Can you work these out from the model? Positions are in its coordinate system, mm. A direction names the side the tool comes from. Coordinates: 2 decimals unless noted, no trailing zeros. Order: outer loops, then holes, each group sorted by start corner. A loop starts at its lowest first (then second) coordinate and runs counter-clockwise, first axis right, second up. Notation, with made-up numbers: (-38.5, 15) -> (-26.5, 15) arc R15 cw to (-26.5, 32) -> close; hole circle Ø7 at (-23, -30). An arc over 180 degrees is marked (long way). Answer in a Markdown table with one row per item.
```python
from build123d import *

# Parameters (mm, degrees)
BOSS_EXTRUDE1_DEPTH = 45
SKETCH3_W           = 92.200496998
SKETCH3_H           = 5.5
BOSS_EXTRUDE2_DEPTH = 1
SKETCH4_R           = 2.5
CUT_EXTRUDE2_DEPTH  = 7.222605
SKETCH8_R           = 4.5
CUT_EXTRUDE7_DEPTH  = 0.386255
CUT_EXTRUDE3_START  = -13.60831
SKETCH5_R           = 2.5
CUT_EXTRUDE3_DEPTH  = 13.60831
CUT_EXTRUDE5_START  = -14
SKETCH6_R           = 4.25
CUT_EXTRUDE5_DEPTH  = 1.7
SKETCH10_R          = 2.6
CUT_EXTRUDE8_DEPTH  = 32
SKETCH11_R          = 10
BOSS_EXTRUDE3_DEPTH = 1
CUT_EXTRUDE10_DEPTH = 46.0000001


with BuildPart() as part:
    # Sketch1 → Boss-Extrude1 (new body)
    with BuildSketch(Plane(origin=(0, 0, 0), x_dir=(1, 0, 0), z_dir=(0, 1, 0))):
        with BuildLine():
            Line((67.073634163, -66.174942219), (25, 6.698729811))
            Line((25, 6.698729811), (43.49555567, 17.377143855))
            ThreePointArc((43.49555567, 17.377143855), (0, 32), (-43.49555567, 17.377143855))
            Line((-43.49555567, 17.377143855), (-25, 6.698729811))
            Line((-25, 6.698729811), (-67.073634163, -66.174942219))
            Line((-67.073634163, -66.174942219), (-71.100248499, -73.149242831))
            Line((-71.100248499, -73.149242831), (-63.915003714, -73.149242831))
            Line((-63.915003714, -73.149242831), (-48.529056191, -46.5))
            ThreePointArc((-48.529056191, -46.5), (-46.698929172, -44.669872981), (-44.198929172, -44))
            Line((-44.198929172, -44), (44.198929172, -44))
            ThreePointArc((44.198929172, -44), (46.698929172, -44.669872981), (48.529056191, -46.5))
            Line((48.529056191, -46.5), (63.915003714, -73.149242831))
            Line((63.915003714, -73.149242831), (71.100248499, -73.149242831))
            Line((71.100248499, -73.149242831), (67.073634163, -66.174942219))
        make_face()
        Polygon((-20, 20), (-13, 20), (-13, 18), (-7, 18), (-7, 20), (7, 20), (7, 18), (13, 18), (13, 20), (20, 20), (20, 13), (18, 13), (18, 7), (20, 7), (20, 0), (-20, 0), (-20, 7), (-18, 7), (-18, 13), (-20, 13), align=None, mode=Mode.SUBTRACT)
        with BuildLine():
            Line((-27.744446501, -15.5), (27.744446501, -15.5))
            ThreePointArc((27.744446501, -15.5), (30.244446501, -16.169872981), (32.074573519, -18))
            Line((32.074573519, -18), (39.580127019, -31))
            ThreePointArc((39.580127019, -31), (39.580127019, -36), (35.25, -38.5))
            Line((35.25, -38.5), (-35.25, -38.5))
            ThreePointArc((-35.25, -38.5), (-39.580127019, -36), (-39.580127019, -31))
            Line((-39.580127019, -31), (-32.074573519, -18))
            ThreePointArc((-32.074573519, -18), (-30.244446501, -16.169872981), (-27.744446501, -15.5))
        make_face(mode=Mode.SUBTRACT)
    extrude(amount=BOSS_EXTRUDE1_DEPTH)

    # Sketch3 → Boss-Extrude2 (add)
    with BuildSketch(Plane(origin=(21.650635095, 0, -12.5), x_dir=(-0.5, 0, -0.866025404), z_dir=(0.866025404, 0, -0.5))):
        with Locations((-52.79897831, 32.25)):
            Rectangle(SKETCH3_W, SKETCH3_H)
        with Locations((-52.79897831, 12.75)):
            Rectangle(SKETCH3_W, SKETCH3_H)
    boss_extrude2 = extrude(amount=BOSS_EXTRUDE2_DEPTH)

    # Sketch4 → Cut-Extrude2 (cut)
    with BuildSketch(Plane(origin=(22.516660498, 0, -13), x_dir=(-0.5, 0, -0.866025404), z_dir=(0.866025404, 0, -0.5))):
        with Locations((-34.198729811, 32.25)):
            Circle(SKETCH4_R)
        with Locations((-34.198729811, 12.75)):
            Circle(SKETCH4_R)
        with Locations((-81.698729811, 12.75)):
            Circle(SKETCH4_R)
        with Locations((-81.698729811, 32.25)):
            Circle(SKETCH4_R)
    cut_extrude2 = extrude(amount=-CUT_EXTRUDE2_DEPTH, mode=Mode.SUBTRACT)

    # Sketch8 → Cut-Extrude7 (cut)
    with BuildSketch(Plane(origin=(16.261701506, 0, -9.388697742), x_dir=(0.5, 0, 0.866025404), z_dir=(-0.866025404, 0, 0.5))):
        with Locations((34.198729811, 32.25)):
            Circle(SKETCH8_R)
        with Locations((34.198729811, 12.75)):
            Circle(SKETCH8_R)
    cut_extrude7 = extrude(amount=CUT_EXTRUDE7_DEPTH, mode=Mode.SUBTRACT)

    # Sketch5 → Cut-Extrude3 (cut)
    with BuildSketch(Plane.XY.offset(-18).offset(CUT_EXTRUDE3_START)):
        with Locations((10, 32.5)):
            Circle(SKETCH5_R)
        with Locations((10, 12.5)):
            Circle(SKETCH5_R)
    cut_extrude3 = extrude(amount=CUT_EXTRUDE3_DEPTH, mode=Mode.SUBTRACT)

    # Sketch6 → Cut-Extrude5 (cut)
    with BuildSketch(Plane.XY.offset(-18).offset(CUT_EXTRUDE5_START)):
        with Locations((10, 32.5)):
            Circle(SKETCH6_R)
        with Locations((10, 12.5)):
            Circle(SKETCH6_R)
    cut_extrude5 = extrude(amount=CUT_EXTRUDE5_DEPTH, mode=Mode.SUBTRACT)

    # Mirror1: Boss-Extrude2, Cut-Extrude2, Cut-Extrude7, Cut-Extrude3, Cut-Extrude5 across plane
    add(boss_extrude2.mirror(Plane(origin=(0, 0, 0), x_dir=(0, 0, 1), z_dir=(1, 0, 0))))
    add(cut_extrude2.mirror(Plane(origin=(0, 0, 0), x_dir=(0, 0, 1), z_dir=(1, 0, 0))), mode=Mode.SUBTRACT)
    add(cut_extrude7.mirror(Plane(origin=(0, 0, 0), x_dir=(0, 0, 1), z_dir=(1, 0, 0))), mode=Mode.SUBTRACT)
    add(cut_extrude3.mirror(Plane(origin=(0, 0, 0), x_dir=(0, 0, 1), z_dir=(1, 0, 0))), mode=Mode.SUBTRACT)
    add(cut_extrude5.mirror(Plane(origin=(0, 0, 0), x_dir=(0, 0, 1), z_dir=(1, 0, 0))), mode=Mode.SUBTRACT)

    # Sketch9 → Revolve1 (revolve)
    with BuildSketch(Plane(origin=(0, 0, 0), x_dir=(0, 0, -1), z_dir=(1, 0, 0))):
        Polygon((-31.1, 26.1), (-31.1, 22.5), (-38.5, 22.5), (-38.5, 37.5), align=None)
        Polygon((-22.9, 26.1), (-15.5, 37.5), (-15.5, 22.5), (-22.9, 22.5), align=None)
    revolve(axis=Axis((0, 22.5, 15.5), (0, 0, 1)))

    # Sketch10 → Cut-Extrude8 (cut)
    with BuildSketch(Plane.XY.offset(44)):
        with Locations((0, 22.5)):
            Circle(SKETCH10_R)
    extrude(amount=-CUT_EXTRUDE8_DEPTH, mode=Mode.SUBTRACT)

    # Sketch11 → Boss-Extrude3 (add)
    with BuildSketch(Plane(origin=(0, 0, 0), x_dir=(1, 0, 0), z_dir=(0, 1, 0))):
        with Locations((62.338794406, -63.196563711)):
            Circle(SKETCH11_R)
        with Locations((-62.338794406, -63.196563711)):
            Circle(SKETCH11_R)
    extrude(amount=BOSS_EXTRUDE3_DEPTH)

    # Sketch14 → Cut-Extrude10 (cut, through all)
    with BuildSketch(Plane(origin=(0, 0, 0), x_dir=(1, 0, 0), z_dir=(0, 1, 0))):
        Polygon((-80, -75.149242831), (80, -75.149242831), (80, -53.149242831), (70, -53.149242831), (70, -69.917804932), (69.425932718, -70.249242831), (-69.425932718, -70.249242831), (-70, -69.917804932), (-70, -53.149242831), (-80, -53.149242831), align=None)
    extrude(amount=CUT_EXTRUDE10_DEPTH, mode=Mode.SUBTRACT)


solid = part.part
```
(1) Will these pins go through, and if not, where does the flat tip stop? pin 1 Ø1.6 at (y, z) = (14.5, -19.5) entering from +X; pin 2 Ø10 at (x, y) = (-10, 32.5) entering from +Z; pin 3 Ø3 at (y, z) = (33, -2.5) entering from +X.
Response values:
| item | result |
|---|---|
| pin 1 | x = 41.69 |
| pin 2 | z = 44 |
| pin 3 | x = 29.44 |
(2) Suppose I cut it at D-D (y = 4.5). Count the separate pieces of the cut face and the enclosed holes in it, and give its area (3 significant figures).
Response values:
| item | result |
|---|---|
| separate pieces | 1 |
| enclosed holes | 2 |
| area | 3,570 mm2 |
(3) On a 3-axis mill with a long thin cutter (end or side, diameter ignored), from which of +Z, -Z, +X, -X, +Y, -Y can I reach the whole of each face in a straight line? I mean faces 4 (the flat face through (-48.242, 12.788, 31.558)), 5 (the flat face through (48, 15.5, 32)), 6 (the flat face through (2, 20, 22.9)), 7 (the flat face through (-48, 10, 32)), 8 (the flat face through (13, 33, -30.3)). Say none if no direction works.
Response values:
| item | result |
|---|---|
| face 4 | -X, +Y |
| face 5 | +X |
| face 6 | +Y, -Y |
| face 7 | -X |
| face 8 | -Z |
(4) We'd pull the mould along Z, two halves only. Please class faces 1 (the flat face through (-9.9, 9.7, -30.3)), 2 (the flat face through (2, 25, 31.1)), 3 (the cylindrical face through (-0.338, 25.078, 17.526)): +Z half, -Z half, draft (parallel to the pull), parting line (faces both ways), or undercut.
Response values:
| item | result |
|---|---|
| face 1 | -Z half |
| face 2 | undercut |
| face 3 | draft |
(5) Suppose I cut it at C-C (x = -23). Please give me the cut outline in (y, z), and give its area (3 significant figures).
Response values:
| item | result |
|---|---|
| outline | (0, -28.23) -> (45, -28.23) -> (45, 15.5) -> (0, 15.5) -> close; (0, 38.5) -> (45, 38.5) -> (45, 44) -> (0, 44) -> close |
| area | 2,220 mm2 |
(6) Suppose I cut it at A-A (x = 0). Please give me the cut outline in (y, z).
Response values:
| item | result |
|---|---|
| outline | (0, -32) -> (45, -32) -> (45, -20) -> (0, -20) -> close; (0, 0) -> (45, 0) -> (45, 15.5) -> (37.5, 15.5) -> (26.1, 22.9) -> (25.1, 22.9) -> (25.1, 12) -> (19.9, 12) -> (19.9, 22.9) -> (18.9, 22.9) -> (7.5, 15.5) -> (0, 15.5) -> close; (0, 38.5) -> (7.5, 38.5) -> (18.9, 31.1) -> (19.9, 31.1) -> (19.9, 44) -> (0, 44) -> close; (25.1, 31.1) -> (26.1, 31.1) -> (37.5, 38.5) -> (45, 38.5) -> (45, 44) -> (25.1, 44) -> close |
(7) Suppose I cut it at B-B (z = 34). Please give me the cut outline in (x, y), and give its area (3 significant figures).
Response values:
| item | result |
|---|---|
| outline | (-49.65, 10) -> (-48.5, 10) -> (-48.5, 0) -> (-40.22, 0) -> (-40.22, 45) -> (-48.5, 45) -> (-48.5, 35) -> (-49.65, 35) -> (-49.65, 29.5) -> (-48.5, 29.5) -> (-48.5, 15.5) -> (-49.65, 15.5) -> close; circle Ø16.14 at (0, 22.5); (40.22, 0) -> (48.5, 0) -> (48.5, 10) -> (49.65, 10) -> (49.65, 15.5) -> (48.5, 15.5) -> (48.5, 29.5) -> (49.65, 29.5) -> (49.65, 35) -> (48.5, 35) -> (48.5, 45) -> (40.22, 45) -> close; hole circle Ø5.2 at (0, 22.5) |
| area | 953 mm2 |
(8) I need wall thicknesses on line 1 (Z direction, x = -16.5, y = 4); line 2 (Z direction, x = -28, y = 12); line 3 (X direction, y = 19, z = 34). Which ranges of each line are inside material? Lowest first, please. Write a range as [from, to].
Response values:
| item | result |
|---|---|
| line 1 | [-30.08, -20], [0, 15.5], [38.5, 44] |
| line 2 | [-26.33, -8.43], [-3.5, 15.51], [38.5, 44] |
| line 3 | [-48.5, -40.22], [-7.27, 7.27], [40.22, 48.5] |
